Part print with two shaded views. Sizes in mm from the minimum x, y, z corner. A direction names the side the tool comes from. Give positions to 0.01 mm unless a question says otherwise; leave off trailing zeros. Write each loop counter-clockwise with the first axis right and the second up, starting at its lowest first coordinate (ties: lowest second). Pieces come first, ordered by that corner, then holes.
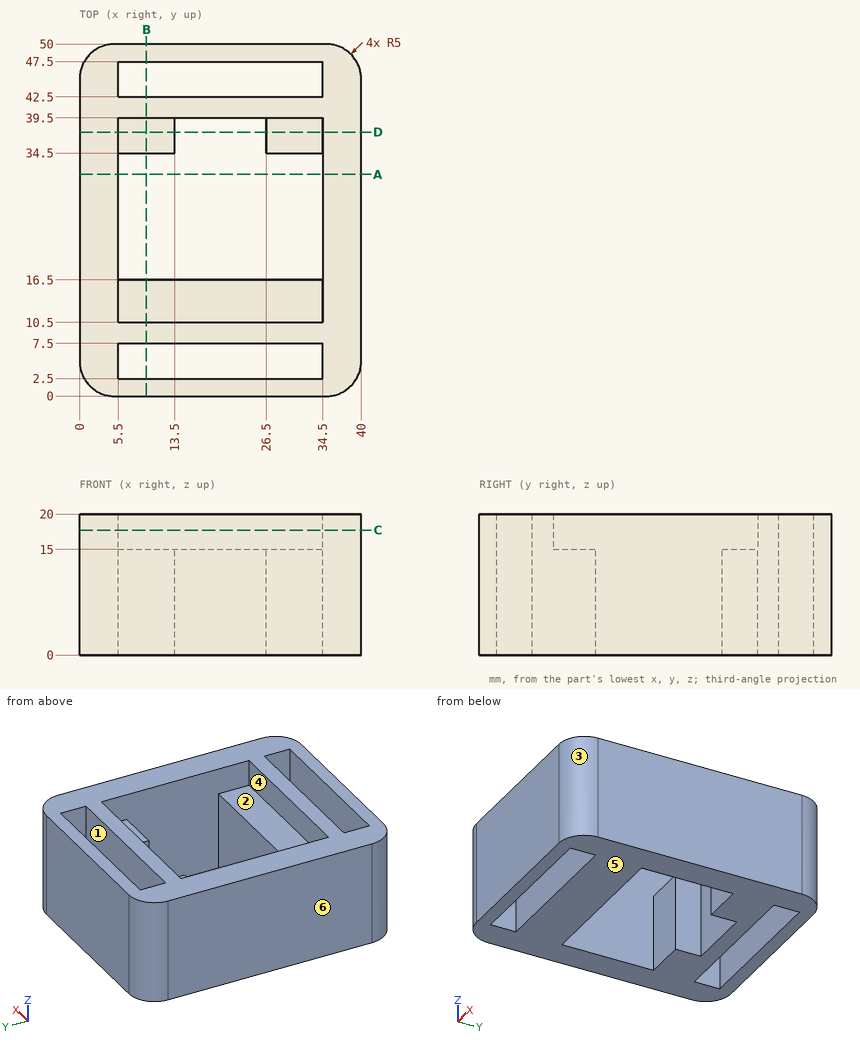
1) Saw through at D-D (y = 37.5). Write the cut outline in (x, z).
Check result:
outline: (0, 0) - (13.5, 0) - (13.5, 15) - (5.5, 15) - (5.5, 20) - (0, 20) - close; (26.5, 0) - (40, 0) - (40, 20) - (34.5, 20) - (34.5, 15) - (26.5, 15) - close
2) Drill centre lines: L1, parallel to Y at x = 20, z = 18.75; L2, parallel to Y at x = 9, z = 14.5; L3, parallel to X at y = 21.5, z = 17.25. Where is each one in solid material? Low to high.
Check result:
L1: y = 0 to 2.5, 7.5 to 10.5, 39.5 to 42.5, 47.5 to 50
L2: y = 0 to 2.5, 7.5 to 16.5, 34.5 to 42.5, 47.5 to 50
L3: x = 0 to 5.5, 34.5 to 40
3) Saw through at A-A (y = 31.5). Write the cut outline in (x, z), and give its area (3 significant figures).
Check result:
outline: (0, 0) - (5.5, 0) - (5.5, 20) - (0, 20) - close; (34.5, 0) - (40, 0) - (40, 20) - (34.5, 20) - close
area: 220 mm2
4) Saw through at B-B (x = 9.5). Write the cut outline in (y, z), and give its area (3 significant figures).
Check result:
outline: (0, 0) - (2.5, 0) - (2.5, 20) - (0, 20) - close; (7.5, 0) - (16.5, 0) - (16.5, 15) - (10.5, 15) - (10.5, 20) - (7.5, 20) - close; (34.5, 0) - (42.5, 0) - (42.5, 20) - (39.5, 20) - (39.5, 15) - (34.5, 15) - close; (47.5, 0) - (50, 0) - (50, 20) - (47.5, 20) - close
area: 385 mm2
5) Mould opens along X. For the marked faces 4, 5 and 6 say: +X half, -X half, draft (parallel to the pull), parting line (faces both ways), or undercut.
Check result:
face 4: undercut
face 5: draft
face 6: -X half
6) Flat gauge pin, fed straight in: P1, Ø2.5, axis at x = 9.5, y = 37.5, coming from the +Z side. Where does the tip first touch, or does it go through?
Check result:
P1: stops at z = 15
7) Saw through at C-C (z = 17.75). Write the cut outline in (x, y), and give its area (3 significant figures).
Check result:
outline: (0, 5) arc R5 ccw to (5, 0) - (35, 0) arc R5 ccw to (40, 5) - (40, 45) arc R5 ccw to (35, 50) - (5, 50) arc R5 ccw to (0, 45) - close; hole (5.5, 2.5) - (34.5, 2.5) - (34.5, 7.5) - (5.5, 7.5) - close; hole (5.5, 10.5) - (34.5, 10.5) - (34.5, 39.5) - (5.5, 39.5) - close; hole (5.5, 42.5) - (34.5, 42.5) - (34.5, 47.5) - (5.5, 47.5) - close
area: 848 mm2
8) 3-axis set-ups, long thin cutter, end or side, ignore diameter. For the marked faces 1, 2 and 3: which of +Z, -Z, +X, -X, +Y, -Y reach the whole face in a straight line?
Check result:
face 1: +Z, -Z
face 2: +Z
face 3: +Z, -Z, +X, -Y
